from build123d import *

# Parameters (mm, degrees)
ESQUISSE1_R             = 11.3
BOSS_EXTRU_1_DEPTH      = 16.5
ESQUISSE2_R             = 4.7
ENL_V_MAT_EXTRU_1_DEPTH = 1.5
ESQUISSE3_R             = 2.6
ENL_V_MAT_EXTRU_2_DEPTH = 3
ENL_V_MAT_EXTRU_3_DEPTH = 6
ESQUISSE5_R             = 1.6
ENL_V_MAT_EXTRU_4_DEPTH = 6.5
ESQUISSE6_W             = 5.85
ESQUISSE6_H             = 2.25
ENL_V_MAT_EXTRU_5_DEPTH = 8
ENL_V_START             = -3.1
ESQUISSE7_R             = 1.6
ENL_V_MAT_EXTRU_6_DEPTH = 28.74345755
ESQUISSE8_R             = 11.3
ENL_V_MAT_EXTRU_7_DEPTH = 23.970198254
ESQUISSE9_R             = 3
ENL_V_MAT_EXTRU_8_DEPTH = 1.2


with BuildPart() as part:
    # Esquisse1 → Boss.-Extru.1 (new body)
    with BuildSketch(Plane(origin=(0, 0, 0), x_dir=(1, 0, 0), z_dir=(0, 1, 0))):
        with Locations(Location((0, 0, 0), (0, 0, 270))):
            Circle(ESQUISSE1_R)
    extrude(amount=BOSS_EXTRU_1_DEPTH)

    # Esquisse2 → Enlèv. mat.-Extru.1 (cut)
    with BuildSketch(Plane.XZ):
        with Locations(Location((0, 0, 0), (0, 0, 270))):
            Circle(ESQUISSE2_R)
    extrude(amount=-ENL_V_MAT_EXTRU_1_DEPTH, mode=Mode.SUBTRACT)

    # Esquisse3 → Enlèv. mat.-Extru.2 (cut)
    with BuildSketch(Plane.XZ.offset(-1.5)):
        with Locations(Location((0, 0, 0), (0, 0, 270))):
            Circle(ESQUISSE3_R)
    extrude(amount=-ENL_V_MAT_EXTRU_2_DEPTH, mode=Mode.SUBTRACT)

    # Esquisse4 → Enlèv. mat.-Extru.3 (cut)
    with BuildSketch(Plane.XZ.offset(-4.5)):
        with BuildLine():
            Line((2.00935313, 1.65), (-2.00935313, 1.65))
            ThreePointArc((-2.00935313, 1.65), (-2.6, 0), (-2.00935313, -1.65))
            Line((-2.00935313, -1.65), (2.00935313, -1.65))
            ThreePointArc((2.00935313, -1.65), (2.447888696, -0.876265332), (2.6, 0))
            ThreePointArc((2.6, 0), (2.447888696, 0.876265332), (2.00935313, 1.65))
        make_face()
    extrude(amount=-ENL_V_MAT_EXTRU_3_DEPTH, mode=Mode.SUBTRACT)

    # Esquisse5 → Enlèv. mat.-Extru.4 (cut)
    with BuildSketch(Plane(origin=(0, 16.5, 0), x_dir=(1, 0, 0), z_dir=(0, 1, 0))):
        with Locations(Location((0, 0, 0), (0, 0, 270))):
            Circle(ESQUISSE5_R)
    extrude(amount=-ENL_V_MAT_EXTRU_4_DEPTH, mode=Mode.SUBTRACT)

    # Esquisse6 → Enlèv. mat.-Extru.5 (cut)
    with BuildSketch(Plane(origin=(0, 16.5, 0), x_dir=(1, 0, 0), z_dir=(0, 1, 0))):
        with Locations((0, -4.225)):
            Rectangle(ESQUISSE6_W, ESQUISSE6_H)
    enl_v_mat_extru_5 = extrude(amount=-ENL_V_MAT_EXTRU_5_DEPTH, mode=Mode.SUBTRACT)

    # Esquisse7 → Enlèv. mat.-Extru.6 (cut)
    with BuildSketch(Plane.XY.offset(3.1).offset(ENL_V_START)):
        with Locations(Location((0, 12.5, 0), (0, 0, 90))):
            Circle(ESQUISSE7_R)
    enl_v_mat_extru_6 = extrude(amount=ENL_V_MAT_EXTRU_6_DEPTH, mode=Mode.SUBTRACT)

    # Esquisse8 → Enlèv. mat.-Extru.7 (cut, through all)
    with BuildSketch(Plane(origin=(0, 16.5, 0), x_dir=(1, 0, 0), z_dir=(0, 1, 0))):
        Circle(ESQUISSE8_R)
        with BuildLine():
            Line((-3.459768778, -8.2), (3.459768778, -8.2))
            ThreePointArc((3.459768778, -8.2), (8.9, 0), (3.459768778, 8.2))
            Line((3.459768778, 8.2), (-3.459768778, 8.2))
            ThreePointArc((-3.459768778, 8.2), (-8.9, 0), (-3.459768778, -8.2))
        make_face(mode=Mode.SUBTRACT)
    extrude(amount=-ENL_V_MAT_EXTRU_7_DEPTH, mode=Mode.SUBTRACT)

    # Esquisse9 → Enlèv. mat.-Extru.8 (cut)
    with BuildSketch(Plane.XY.offset(8.2)):
        with Locations((0, 12.5)):
            Circle(ESQUISSE9_R)
    enl_v_mat_extru_8 = extrude(amount=-ENL_V_MAT_EXTRU_8_DEPTH, mode=Mode.SUBTRACT)

    # Symétrie1: Enlèv. mat.-Extru.5, Enlèv. mat.-Extru.6, Enlèv. mat.-Extru.8 across plane
    add(enl_v_mat_extru_5.mirror(Plane.XY), mode=Mode.SUBTRACT)
    add(enl_v_mat_extru_6.mirror(Plane.XY), mode=Mode.SUBTRACT)
    add(enl_v_mat_extru_8.mirror(Plane.XY), mode=Mode.SUBTRACT)


solid = part.part
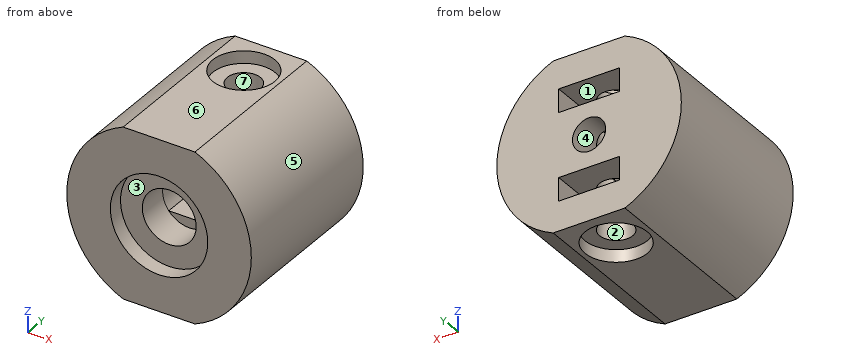
Geometry: final body of the model. Coordinates: model frame, mm. Face numbers are marked on the shaded views. A direction names the side the tool comes from. Coordinates: 2 decimals unless noted, no trailing zeros. Loops run counter-clockwise (first coordinate to the right, second up) from the corner with the lowest first, then second, coordinate; pieces in that order, holes last. Notation, with made-up numbers: (-34, 39.25) - (5, 39.25) arc R30 ccw to (5, 76.25) - close; hole circle Ø11 at (-11, 50.5). An arc over 180 degrees is marked (long way). Put each result on its own line as item: value. Start each with the question number.
Q1. Cut plane B-B, the plane z = 4. Return loops of the section in (x, y) (3 decimals).
Q2. Cut plane A-A, the plane y = 7.25. Return loops of the section in (x, z), and give its area (3 significant figures).
Q3. Cut plane D-D, the plane z = -3.75. Return loops of the section in (x, y) (3 decimals), and give its area (3 significant figures).
Q4. Cut plane C-C, the plane x = 0. Give the number of separate pieces and of enclosed holes in the cut face, and give its area (3 significant figures).
Q5. Line query: line 1 (Y direction, x = 0, z = -7.7); line 2 (X direction, y = 1.25, z = 0); line 3 (X direction, y = 13.75, z = 0). Output: solid intervals per line, ascending.
Q6. Pull-direction query (Z, two-part tool) for the marked faces 4, 5, 6 and 7; classes: released by +Z, released by -Z, zero draft, split by the parting line, or undercut.
Q7. Set-up query: the marked faces 1, 2 and 3. Return all of +Z, -Z, +X, -X, +Y, -Y with unobstructed straight access to the full face (end or side cutting, diameter ignored); none if empty.
Q8. Pin query (flat end, axial travel): pin 1 Ø4 at (x, y) = (0, 12.5) entering from -Z; pin 2 Ø0.7 at (x, z) = (-0.5, -4.5) entering from +Y; pin 3 Ø2.5 at (y, z) = (12, 4.5) entering from -X. Return the tip coordinate at first contact, or that it passes through.
Filled sheet:
1. outline: (-7.95, 0) - (-2.468, 0) - (-2.468, 1.5) - (2.468, 1.5) - (2.468, 0) - (7.95, 0) - (7.95, 16.5) - (2.925, 16.5) - (2.925, 8.5) - (-2.925, 8.5) - (-2.925, 16.5) - (-7.95, 16.5) - close
2. outline: (-3.46, -8.2) - (3.46, -8.2) arc R8.9 ccw to (3.46, 8.2) - (-3.46, 8.2) arc R8.9 ccw to start; hole (-2.01, -1.65) - (2.01, -1.65) arc R2.6 ccw to (2.01, 1.65) - (-2.01, 1.65) arc R2.6 ccw to start
2. area: 226 mm²
3. outline: (-8.071, 0) - (-2.833, 0) - (-2.833, 1.5) - (2.833, 1.5) - (2.833, 0) - (8.071, 0) - (8.071, 16.5) - (2.925, 16.5) - (2.925, 8.5) - (-2.925, 8.5) - (-2.925, 16.5) - (-8.071, 16.5) - close
3. area: 211 mm²
4. separate pieces: 6
4. enclosed holes: 0
4. area: 131 mm²
5. line 1: 0 to 9.5, 15.5 to 16.5
5. line 2: -8.9 to -4.7, 4.7 to 8.9
5. line 3: -8.9 to -1.6, 1.6 to 8.9
6. face 4: undercut
6. face 5: split by the parting line
6. face 6: released by +Z
6. face 7: zero draft
7. face 1: +Y
7. face 2: +Z, -Z
7. face 3: -Y
8. pin 1: z = -7
8. pin 2: y = 8.5
8. pin 3: x = -8.29
